Autodesk Inventor part; units mm, degrees
ref_plane "YZ Plane" through (0, 0, 0) normal (1, 0, 0) x (0, 1, 0)
ref_plane "XZ Plane" through (0, 0, 0) normal (0, 1, 0) x (-1, 0, 0)
ref_plane "XY Plane" through (0, 0, 0) normal (0, 0, 1) x (1, 0, 0)
sketch "Sketch1" plane through (0, 0, 0) normal (0, 1, 0) x (-1, 0, 0)
  line L0 (-44.45, -52.3875) -> (44.45, -52.3875)
  line L1 (44.45, -52.3875) -> (44.45, 52.3875)
  line L2 (44.45, 52.3875) -> (-44.45, 52.3875)
  line L3 (-44.45, 52.3875) -> (-44.45, -52.3875)
  line L4 (-44.45, -52.3875) -> (44.45, 52.3875) construction
  line L5 (44.45, -52.3875) -> (-44.45, 52.3875) construction
  point P0 (0, 0)
  dimension "d0" = 104.775
  dimension "d1" = 88.9
extrude "Extrusion1" add sketch "Sketch1" along normal blind 12.7
sketch "Sketch2" plane through (0, 12.7, 0) normal (0, 1, 0) x (1, 0, 0)
  line L0 (44.45, 52.3875) -> (-44.45, 52.3875)
  line L1 (-44.45, 52.3875) -> (-44.45, -52.3875)
  line L2 (44.45, 52.3875) -> (-44.45, 52.3875)
  line L3 (-44.45, 52.3875) -> (-44.45, -52.3875)
  line L4 (-44.45, -52.3875) -> (44.45, -52.3875)
  line L5 (44.45, -52.3875) -> (44.45, 52.3875)
  point P0 (0, 0)
  dimension "d4" = 104.775
extrude "Extrusion2" add sketch "Sketch2" along normal blind 38.1
sketch "Sketch4" plane through (-44.45, 0, -52.3875) normal (-1, 0, 0) x (0, 0, 1)
  line L0 (101.6, 47.625) -> (3.175, 47.625)
  line L1 (3.175, 47.625) -> (3.175, 12.7)
  line L2 (3.175, 12.7) -> (101.6, 12.7)
  line L3 (101.6, 12.7) -> (101.6, 47.625)
  line L4 (0, 0) -> (0, 50.8)
  line L5 (0, 50.8) -> (104.775, 50.8)
  line L6 (104.775, 12.7) -> (104.775, 50.8)
  line L7 (0, 0) -> (104.775, 0)
  point P0 (52.3875, 0)
  dimension "d11" = 3.175
  dimension "d12" = 3.175
  dimension "d14" = 12.7
  dimension "d33" = 3.175
extrude "Extrusion3" cut sketch "Sketch4" against normal blind 85.725
sketch "Sketch5" plane through (0, 50.8, 0) normal (0, 1, 0) x (1, 0, 0)
  line L0 (-44.45, 52.3875) -> (-44.45, -52.3875)
  line L1 (44.45, -52.3875) -> (44.45, 52.3875)
  line L2 (-44.45, -39.6875) -> (44.45, -39.6875)
  line L3 (44.45, -39.6875) -> (44.45, 39.6875)
  line L4 (44.45, 39.6875) -> (-44.45, 39.6875)
  line L5 (-44.45, 39.6875) -> (-44.45, -39.6875)
  line L6 (44.45, 52.3875) -> (-44.45, 52.3875)
  line L7 (-44.45, -52.3875) -> (44.45, -52.3875)
  point P0 (0, 0)
  dimension "d17" = 12.7
  dimension "d18" = 12.7
extrude "Extrusion4" cut sketch "Sketch5" against normal blind 31.75 contours L4 L1 L2 L0
sketch "Sketch7" plane through (44.45, 0, -52.3875) normal (0, 0, -1) x (-1, 0, 0)
  line L0 (88.9, 0) -> (0, 0)
  line L1 (0, 0) -> (0, 50.8)
  line L2 (88.9, 0) -> (0, 0)
  line L3 (0, 0) -> (0, 12.7)
  line L4 (0, 12.7) -> (88.9, 12.7)
  line L5 (88.9, 12.7) -> (88.9, 0)
  point P0 (44.45, 0)
  dimension "d30" = 12.7
extrude "Extrusion5" add sketch "Sketch7" along normal blind 19.05
sketch "Sketch8" plane through (-44.45, 12.7, -52.3875) normal (0, 1, 0) x (1, 0, 0)
  line L0 (0, 0) -> (0, 19.05)
  line L1 (88.9, 0) -> (88.9, 19.05)
  point P0 (44.45, -52.3875)
  point P1 (19.05, 10.5709)
  point P2 (69.85, 10.5709)
  dimension "d34" = 50.8
  dimension "d36" = 19.05
hole "Hole2" at (-25.4, 12.7, -62.9584) at (25.4, 12.7, -62.9584) direction (0, -1, 0) diameter 6.7564 end through all
properties part number "KVM Holder Left"
Source: CAD feature listing. Evaluate the final solid. Frame: model axes, mm. A direction names the side the tool comes from. Round coordinates to 2 decimals unless told otherwise and drop trailing zeros. Loops run counter-clockwise (first coordinate to the right, second up) from the corner with the lowest first, then second, coordinate; pieces in that order, holes last.
1. Section query A-A on x = -25.4. Output: boundary loops of the cut face in (y, z) (1 decimal).
2. Contact query for flat-ended pins moving along their axis: pin 1 (2.5 mm diameter, centred on x = 43.5, z = -10, fed in from +Y); pin 2 (6 mm diameter, centred on x = -21.5, z = -36, fed in from +Y); pin 3 (4 mm diameter, centred on x = 11, z = -30, fed in from -Y); pin 4 (4 mm diameter, centred on x = -25.4, z = -62.96, fed in from -Y). Output: stop coordinate, or through.
3. Section query C-C on z = -61. Output: boundary loops of the cut face in (x, y), and give its area (3 significant figures).
4. Access query for faces 4 (the flat face through (-2, 30, -49.212)), 5 (the cylindrical face through (-25.549, 6.261, -66.333)), 6 (the flat face through (10, 49, 39.688)), 7 (the flat face through (44.45, 14, -9)), 8 (the flat face through (1, 12.7, -62)). Directions: +Z, -Z, +X, -X, +Y, -Y. A direction counts if a zero-diameter tool reaches every point of the face in a straight line with its end or side. Return the directions, or none.
5. Section query D-D on x = 19. Output: boundary loops of the cut face in (y, z) (1 decimal).
6. Mould query, pull axis Y, two halves, no side actions, for faces 1 (the flat face through (43, 19.05, -1)), 2 (the flat face through (-2, 47.625, -44)), 3 (the cylindrical face through (27.456, 6.261, -65.639)). Classes: released by +Y, released by -Y, zero draft, split by the parting line, or undercut.
7. Ray query, L1, parallel to Y at x = 23.5, z = -42 (3 decimals); L2, parallel to Z at x = 25, y = 9; L3, parallel to Z at x = 7.5, y = 24. Return the intervals inside material, ascending.
Answers below:
1. outline: (0, -71.4) - (12.7, -71.4) - (12.7, -66.3) - (0, -66.3) - close; (0, -59.6) - (12.7, -59.6) - (12.7, -52.4) - (50.8, -52.4) - (50.8, -39.7) - (47.6, -39.7) - (47.6, -49.2) - (12.7, -49.2) - (12.7, 49.2) - (47.6, 49.2) - (47.6, 39.7) - (50.8, 39.7) - (50.8, 52.4) - (0, 52.4) - close
2. pin 1: stops at y = 19.05
2. pin 2: stops at y = 12.7
2. pin 3: stops at y = 0
2. pin 4: passes through
3. outline: (-44.45, 0) - (-28.15, 0) - (-28.15, 12.7) - (-44.45, 12.7) - close; (-22.65, 0) - (22.65, 0) - (22.65, 12.7) - (-22.65, 12.7) - close; (28.15, 0) - (44.45, 0) - (44.45, 12.7) - (28.15, 12.7) - close
3. area: 989 mm2
4. face 4: -X
4. face 5: +Y, -Y
4. face 6: +X, -X, +Y
4. face 7: +Z, -Z, +X, +Y, -Y
4. face 8: -Z, +X, -X, +Y
5. outline: (0, -71.4) - (12.7, -71.4) - (12.7, -52.4) - (50.8, -52.4) - (50.8, -39.7) - (47.6, -39.7) - (47.6, -49.2) - (12.7, -49.2) - (12.7, 49.2) - (47.6, 49.2) - (47.6, 39.7) - (50.8, 39.7) - (50.8, 52.4) - (0, 52.4) - close
6. face 1: released by +Y
6. face 2: undercut
6. face 3: zero draft
7. L1: y = 0 to 12.7, 47.625 to 50.8
7. L2: z = -71.44 to -66.31, -59.6 to 52.39
7. L3: z = -52.39 to -49.21, 49.21 to 52.39
